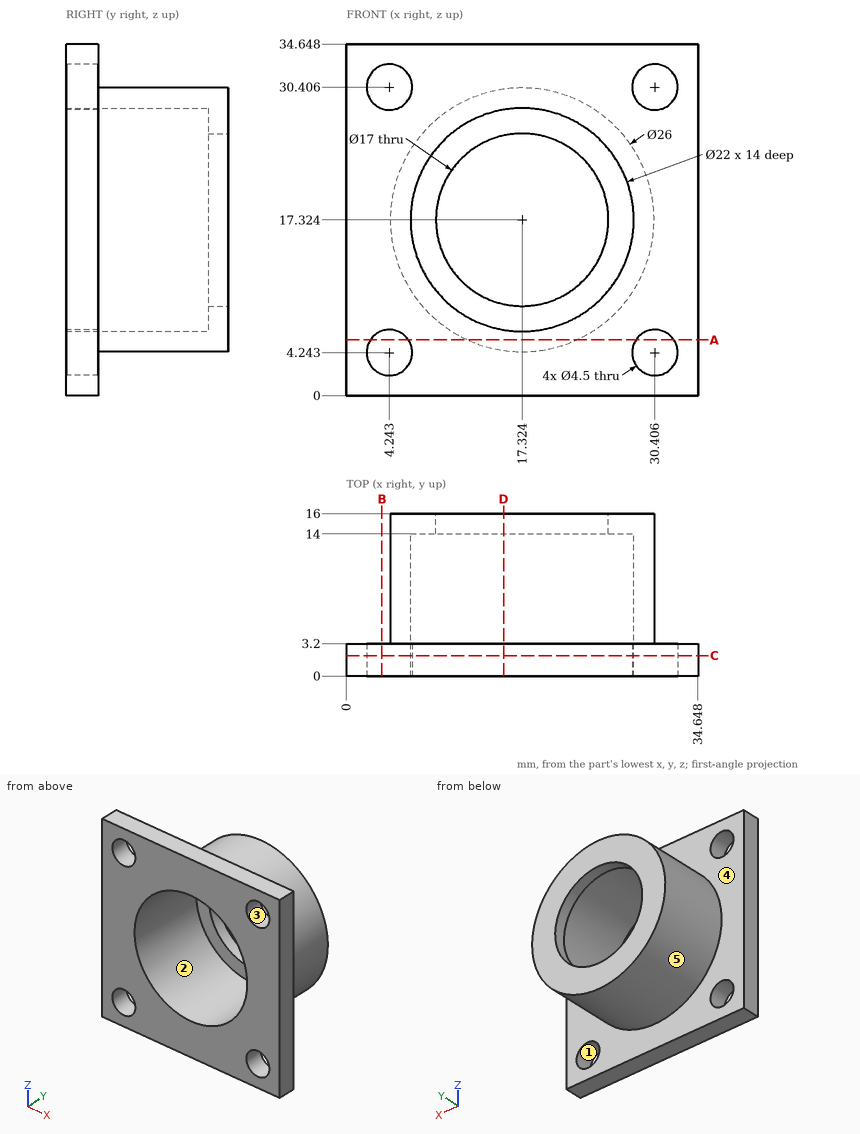
Here's the drawing with two shaded views (mm, measured from the low corner). I have some questions. A direction names the side the tool comes from. Round coordinates to 2 decimals unless told otherwise and drop trailing zeros. Order: outer loops, then holes, each group sorted by start corner. A loop starts at its lowest first (then second) coordinate and runs counter-clockwise, first axis right, second up. Notation, with made-up numbers: (41.25, 59) -> (74.25, 59) arc R30 cw to (74.25, 94) -> close; hole circle Ø7 at (53, 79.5). An arc over 180 degrees is marked (long way). Use a Markdown table: item, result. Add a question column.
(1) Suppose I cut it at C-C, the plane y = 2. Count the separate pieces of the cut face and the enclosed holes in it, and give its area (3 significant figures).
(2) I need wall thicknesses on line 1 along Y through (x, z) = (24, 25.5); line 2 along X through (y, z) = (4.75, 8) (1 decimal); line 3 along Z through (x, y) = (11.5, 15.5) (1 decimal). Which ranges of each line are inside material? Lowest first, please.
(3) If we mould it in two halves opening along X, with no side actions, what happens to the marked faces 3, 4 and 5? For each: released by +X, released by -X, zero draft, split by the parting line, or undercut.
(4) For pin 1 Ø6 at (x, z) = (30.41, 30.41) entering from +Y; pin 2 Ø15.5 at (x, z) = (17.32, 17.32) entering from +Y; pin 3 Ø11 at (x, z) = (12.5, 18) entering from -Y; pin 4 Ø2 at (x, y) = (24.5, 8) entering from -Z (1 decimal), each with a flat end and sliding along its axis, tell me the tip position at first contact or that it passes through.
(5) For the marked faces 1 and 2, which set-ups out of +Z, -Z, +X, -X, +Y, -Y let a thin tool reach every point of the face, with its end or its side?
(6) Suppose I cut it at D-D, the plane x = 15.5. Please give me the cut outline in (y, z) (1 decimal).
(7) Suppose I cut it at A-A, the plane z = 5.5. Please give me the cut outline in (x, y).
(8) Suppose I cut it at B-B, the plane x = 3.5. Please give me the cut outline in (y, z).
Verdict:
| question | item | result |
|---|---|---|
| 1 | separate pieces | 1 |
| 1 | enclosed holes | 5 |
| 1 | area | 757 mm2 |
| 2 | line 1 | 14 to 16 |
| 2 | line 2 | 8.3 to 11.5, 23.2 to 26.4 |
| 2 | line 3 | 5.7 to 11.1, 23.5 to 28.9 |
| 3 | face 3 | undercut |
| 3 | face 4 | zero draft |
| 3 | face 5 | split by the parting line |
| 4 | pin 1 | y = 3.2 |
| 4 | pin 2 | through |
| 4 | pin 3 | y = 14 |
| 4 | pin 4 | z = 5.9 |
| 5 | face 1 | +Y, -Y |
| 5 | face 2 | -Y |
| 6 | outline | (0, 0) -> (3.2, 0) -> (3.2, 4.5) -> (16, 4.5) -> (16, 9) -> (14, 9) -> (14, 6.5) -> (0, 6.5) -> close; (0, 28.2) -> (14, 28.2) -> (14, 25.6) -> (16, 25.6) -> (16, 30.2) -> (3.2, 30.2) -> (3.2, 34.6) -> (0, 34.6) -> close |
| 7 | outline | (0, 0) -> (2.38, 0) -> (2.38, 3.2) -> (0, 3.2) -> close; (6.11, 0) -> (28.54, 0) -> (28.54, 3.2) -> (22.73, 3.2) -> (22.73, 16) -> (11.92, 16) -> (11.92, 3.2) -> (6.11, 3.2) -> close; (32.27, 0) -> (34.65, 0) -> (34.65, 3.2) -> (32.27, 3.2) -> close |
| 8 | outline | (0, 0) -> (3.2, 0) -> (3.2, 2.12) -> (0, 2.12) -> close; (0, 6.37) -> (3.2, 6.37) -> (3.2, 28.28) -> (0, 28.28) -> close; (0, 32.53) -> (3.2, 32.53) -> (3.2, 34.65) -> (0, 34.65) -> close |
